from build123d import *

# Parameters (mm, degrees)
F0_W     = 25.4
F0_H     = 25.4
F1_DEPTH = 7.366
F3_DEPTH = 7.366


with BuildPart() as f1:
    # F0 (on Top) → F1 (new body)
    with BuildSketch(Plane.XY):
        with Locations((12.7, 12.7)):
            Rectangle(F0_W, F0_H)
    extrude(amount=F1_DEPTH)

    # F2 (on Top) → F3 (join)
    with BuildSketch(Plane.XY):
        with BuildLine():
            Line((5.08, 25.4), (5.08, 31.537144))
            ThreePointArc((5.08, 31.537144), (2.431698, 30.234662), (0, 28.562295))
            Line((0, 28.562295), (0, 25.4))
            Line((0, 25.4), (5.08, 25.4))
        make_face()
        with BuildLine():
            Line((28.562295, 25.4), (25.4, 25.4))
            Line((25.4, 25.4), (25.4, 20.32))
            Line((25.4, 20.32), (31.537144, 20.32))
            ThreePointArc((31.537144, 20.32), (30.234662, 22.968302), (28.562295, 25.4))
        make_face()
        with BuildLine():
            Line((25.4, -3.162295), (25.4, 0))
            Line((25.4, 0), (20.32, 0))
            Line((20.32, 0), (20.32, -6.137144))
            ThreePointArc((20.32, -6.137144), (22.968302, -4.834662), (25.4, -3.162295))
        make_face()
        with BuildLine():
            Line((-3.162295, 0), (0, 0))
            Line((0, 0), (0, 5.08))
            Line((0, 5.08), (-6.137144, 5.08))
            ThreePointArc((-6.137144, 5.08), (-4.834662, 2.431698), (-3.162295, 0))
        make_face()
    extrude(amount=F3_DEPTH)


solid = f1.part
Work out the finished part from the listing and answer in its coordinate system (mm). A direction names the side the tool comes from. Round coordinates to 2 decimals unless told otherwise and drop trailing zeros. Order: outer loops, then holes, each group sorted by start corner. A loop starts at its lowest first (then second) coordinate and runs counter-clockwise, first axis right, second up. Notation, with made-up numbers: M -25.5,12.25 L 31.5,12.25 A13 cw 31.5,19.25 Z; hole C 70,55 d9. An arc over 180 degrees is marked long. Put each result on its own line as item: value. Start each with the question number.
Q1. Straight lines are drawn through the part: L1, parallel to X at y = 13.5, z = 6.5; L2, parallel to Y at x = 27, z = 1.75. For each, find the intervals that lie inside material, in ascending order. Write a range as [from, to].
Q2. Section B-B, the plane y = 11 is taken. Write down the section's boundary in (x, z).
Q3. Flat-ended cylindrical pins translate along their axes: pin 1 (1 mm diameter, centred on y = 0, z = 4.5, fed in from -X); pin 2 (2 mm diameter, centred on x = 12, z = 2.5, fed in from -Y); pin 3 (4 mm diameter, centred on y = 7, z = 6.5, fed in from -X); pin 4 (3 mm diameter, centred on x = 3.5, y = 15.5, fed in from -Z). Find the tip coordinate at first contact, or state that the pin passes through.
Q4. A tool of negligible diameter and unlimited length cuts with its end or side. For faces 1 (the flat face through (12, 13, 0)), 2 (the flat face through (17, 25.4, 4)), 3 (the flat face through (8, 0, 4)), 4 (the flat face through (-3, 5.08, 4)), 5 (the flat face through (28, 20.32, 4)), from which of +Z, -Z, +X, -X, +Y, -Y can it reach the whole face along a straight path? Write none if from no direction.
Q5. Section C-C, the plane x = -2 is taken. Write down the section's boundary in (y, z), and give its area (3 significant figures).
Q6. Section A-A, the plane z = 3.75 is taken. Write down the section's boundary in (x, y).
Findings below:
1. L1: x = [0, 25.4]
1. L2: y = [20.32, 25.4]
2. outline: M 0,0 L 25.4,0 L 25.4,7.37 L 0,7.37 Z
3. pin 1: stops at x = -3.55
3. pin 2: stops at y = 0
3. pin 3: stops at x = -6.14
3. pin 4: stops at z = 0
4. face 1: -Z, +X, -X, +Y, -Y
4. face 2: +Z, -Z, +X, +Y
4. face 3: +Z, -Z, -X, -Y
4. face 4: +Z, -Z, -X, +Y
4. face 5: +Z, -Z, +X, -Y
5. outline: M 0,0 L 5.08,0 L 5.08,7.37 L 0,7.37 Z
5. area: 37.4 mm^2
6. outline: M -6.14,5.08 A20.32 ccw -3.16,0 L 20.32,0 L 20.32,-6.14 A20.32 ccw 25.4,-3.16 L 25.4,20.32 L 31.54,20.32 A20.32 ccw 28.56,25.4 L 5.08,25.4 L 5.08,31.54 A20.32 ccw 0,28.56 L 0,5.08 Z
